```python
from build123d import *

# Parameters (mm, degrees)
BOSS_EXTRUDE1_DEPTH    = 60
CUT_EXTRUDE1_DEPTH     = 128.644720336
MOVE_START             = 10
MOVE_FACE1_OUTLINE_W   = 23
MOVE_FACE1_OUTLINE_H   = 122
MOVE_FACE1_DEPTH       = 0.1
MOVE_START_2           = 19.9
MOVE_FACE1_2_OUTLINE_W = 23
MOVE_FACE1_2_OUTLINE_H = 122
MOVE_FACE1_2_DEPTH     = 0.1
CHAMFER1_SIZE          = 2.5


# Read off the part's stored shape, not the designer's step: Move Face1
with BuildPart() as part:
    # Sketch1 → Boss-Extrude1 (new, symmetric)
    with BuildSketch(Plane.XY):
        Polygon((0, 38.637033052), (10.352761804, 0), (20.008855708, 2.6), (10.352761804, 38.637033052), align=None)
    extrude(amount=BOSS_EXTRUDE1_DEPTH, both=True)

    # Sketch2 → Cut-Extrude1 (cut, through all)
    with BuildSketch(Plane.XY.offset(60)):
        Polygon((5.176380902, 19.318516526), (14.832474806, 21.918516526), (10.352761804, 38.637033052), (0, 38.637033052), align=None)
    extrude(amount=-CUT_EXTRUDE1_DEPTH, mode=Mode.SUBTRACT)

    # Move Face1 outline → Move Face1 (cut)
    with BuildSketch(Plane(origin=(0, 0, 0), x_dir=(-0.258819045102515, 0.9659258262890698, 0), z_dir=(0.9659258262890699, 0.258819045102515, 0)).offset(MOVE_START)):
        with Locations((7.5, 0)):
            Rectangle(MOVE_FACE1_OUTLINE_W, MOVE_FACE1_OUTLINE_H)
    extrude(amount=MOVE_FACE1_DEPTH, mode=Mode.SUBTRACT)

    # Move Face1 2 outline → Move Face1 2 (cut)
    with BuildSketch(Plane(origin=(0, 0, 0), x_dir=(-0.258819045102515, 0.9659258262890698, 0), z_dir=(0.9659258262890699, 0.258819045102515, 0)).offset(MOVE_START_2)):
        with Locations((7.5, 0)):
            Rectangle(MOVE_FACE1_2_OUTLINE_W, MOVE_FACE1_2_OUTLINE_H)
    extrude(amount=MOVE_FACE1_2_DEPTH, mode=Mode.SUBTRACT)

    # Chamfer1
    chamfer1_edges = [part.edges().sort_by_distance(p)[0] for p in [
        (7.861132292, 9.685258263, -60),
        (7.861132292, 9.685258263, 60),
        (17.324104318, 12.233258263, -60),
        (17.324104318, 12.233258263, 60),
    ]]
    chamfer(chamfer1_edges, length=CHAMFER1_SIZE)


solid = part.part
```
The model under review builds one solid part; all positions refer to its coordinate system, in mm. Round coordinates to 2 decimals unless told otherwise and drop trailing zeros. Order: outer loops, then holes, each group sorted by start corner. A loop starts at its lowest first (then second) coordinate and runs counter-clockwise, first axis right, second up.
(1) Take a section at A-A, the plane z = -23.5. State the section outline as (x, y) points.
Working result:
outline: (5.27, 19.34) - (10.45, 0.03) - (19.91, 2.57) - (14.74, 21.89) - close
(2) For P1, Ø8, axis at x = 7, y = 3, coming from the -Z side; P2, Ø8, axis at y = 9, z = -21, coming from the -X side; P3, Ø4, axis at x = 9, z = 44.5, coming from the +Y side, all flat-tipped, find the tip position at first contact; note any pin that passes through.
Working result:
P1: stops at z = -58.94
P2: stops at x = 6.97
P3: stops at y = 20.89
(3) Wall thickness on L1, parallel to Y at x = 11.5, z = 12; L2, parallel to Y at x = 14.5, z = 52.5; L3, parallel to X at y = 10.5, z = 11: over which ranges is each line inside the solid? List them lowest first.
Working result:
L1: y = 0.31 to 21.02
L2: y = 1.12 to 21.83
L3: x = 7.64 to 17.79
(4) Take a section at B-B, the plane y = 5. State the section outline as (x, z) points.
Working result:
outline: (9.12, -57.5) - (11.7, -60) - (16.67, -60) - (19.26, -57.5) - (19.26, 57.5) - (16.67, 60) - (11.7, 60) - (9.12, 57.5) - close
